from build123d import *

# Parameters (mm, degrees)
SKETCH_1_R          = 1.6
SKETCH_1_R_2        = 3.2
EXTRUDE_1_DEPTH     = 4
SKETCH_2_R          = 3.2
EXTRUDE_2_DEPTH     = 10
CUT_EXTRUDE_1_DEPTH = 10
CUT_EXTRUDE_2_DEPTH = 10


with BuildPart() as part:
    # 草图1 → 凸台-拉伸1 (new body)
    with BuildSketch(Plane.XY):
        Polygon((0, 0), (0, 26), (10, 26), (18, 18), (18, 8), (10, 0), align=None)
        with Locations((5, 21)):
            Circle(SKETCH_1_R, mode=Mode.SUBTRACT)
        with Locations((5, 13)):
            Circle(SKETCH_1_R_2, mode=Mode.SUBTRACT)
        with Locations((5, 5)):
            Circle(SKETCH_1_R, mode=Mode.SUBTRACT)
        with Locations((13, 13)):
            Circle(SKETCH_1_R, mode=Mode.SUBTRACT)
    extrude(amount=EXTRUDE_1_DEPTH)

    # 草图2 → 凸台-拉伸2 (add)
    with BuildSketch(Plane.XY.offset(4)):
        with BuildLine():
            Line((13.468501969, 16.468501969), (16.5, 19.5))
            Line((16.5, 19.5), (11.5, 24.5))
            Line((11.5, 24.5), (8.468501969, 21.468501969))
            ThreePointArc((8.468501969, 21.468501969), (7.104490226, 18.203373302), (3.589329863, 17.796875))
            ThreePointArc((3.589329863, 17.796875), (0, 13), (3.589329863, 8.203125))
            ThreePointArc((3.589329863, 8.203125), (7.104490226, 7.796626698), (8.468501969, 4.531498031))
            Line((8.468501969, 4.531498031), (11.5, 1.5))
            Line((11.5, 1.5), (16.5, 6.5))
            Line((16.5, 6.5), (13.468501969, 9.531498031))
            ThreePointArc((13.468501969, 9.531498031), (9.5, 13), (13.468501969, 16.468501969))
        make_face()
        with Locations((5, 13)):
            Circle(SKETCH_2_R, mode=Mode.SUBTRACT)
    extrude(amount=EXTRUDE_2_DEPTH)

    # 草图3 → 切除-拉伸1 (cut)
    with BuildSketch(Plane(origin=(-1.5, 1.5, 0), x_dir=(0, 0, -1), z_dir=(0.707106781, -0.707106781, 0))):
        Polygon((-4, 25.455844123), (-14, 25.455844123), (-14, 21.168658492), align=None)
    extrude(amount=-CUT_EXTRUDE_1_DEPTH, mode=Mode.SUBTRACT)

    # 草图4 → 切除-拉伸2 (cut)
    with BuildSketch(Plane(origin=(11.5, 11.5, 0), x_dir=(0, 0, -1), z_dir=(0.707106781, 0.707106781, 0))):
        Polygon((-4, -7.071067812), (-14, -2.783882181), (-14, -7.071067812), align=None)
    extrude(amount=-CUT_EXTRUDE_2_DEPTH, mode=Mode.SUBTRACT)


solid = part.part
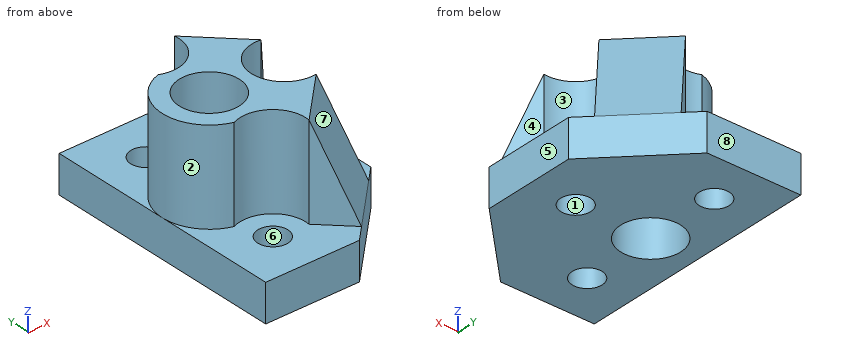
Part model, mm, in its own coordinate system. Face numbers are marked on the shaded views. A direction names the side the tool comes from. Coordinates: 2 decimals unless noted, no trailing zeros. Order: outer loops, then holes, each group sorted by start corner. A loop starts at its lowest first (then second) coordinate and runs counter-clockwise, first axis right, second up.
(1) Probe L1, parallel to Y at x = 5, z = 2; L2, parallel to Y at x = 5, z = 10.5; L3, parallel to Z at x = 10.25, y = 25. List the from-to ranges inside material, lowest first.
Check sheet entries:
L1: y = 0 to 3.4, 6.6 to 9.8, 16.2 to 19.4, 22.6 to 26
L2: y = 8.5 to 9.8, 16.2 to 17.5
L3: z = 0 to 4
(2) Pin check, flat tips, straight feed: pin 1 Ø5 at (x, y) = (13, 13) entering from +Z; pin 2 Ø6 at (x, y) = (5, 13) entering from +Z; pin 3 Ø6 at (x, z) = (15, 5.5) entering from -Y; pin 4 Ø2 at (x, z) = (9.5, 8.5) entering from -Y. Stop position of each tip, or through.
Check sheet entries:
pin 1: stops at z = 4
pin 2: passes through
pin 3: stops at y = 2.4
pin 4: stops at y = 2.69
(3) Slice it at A-A, the plane z = 1.25. Write the cut outline in (x, y).
Check sheet entries:
outline: (0, 0) - (10, 0) - (18, 8) - (18, 18) - (10, 26) - (0, 26) - close; hole circle Ø6.4 at (5, 13); hole circle Ø3.2 at (5, 5); hole circle Ø3.2 at (5, 21); hole circle Ø3.2 at (13, 13)
(4) Slice it at D-D, the plane z = 12.75. Write the cut outline in (x, y).
Check sheet entries:
outline: (3.59, 8.2) arc R3.5 cw to (8.47, 4.53) - (8.85, 4.15) - (13.85, 9.15) - (13.47, 9.53) arc R3.5 cw (long way) to (13.47, 16.47) - (13.85, 16.85) - (8.85, 21.85) - (8.47, 21.47) arc R3.5 cw to (3.59, 17.8) arc R5 ccw to start; hole circle Ø6.4 at (5, 13)
(5) Slice it at B-B, the plane x = 5. Write the cut outline in (y, z).
Check sheet entries:
outline: (0, 0) - (3.4, 0) - (3.4, 4) - (0, 4) - close; (6.6, 0) - (9.8, 0) - (9.8, 14) - (8.5, 14) - (8.5, 4) - (6.6, 4) - close; (16.2, 0) - (19.4, 0) - (19.4, 4) - (17.5, 4) - (17.5, 14) - (16.2, 14) - close; (22.6, 0) - (26, 0) - (26, 4) - (22.6, 4) - close
(6) Pull direction X, two halves, no side cores. Call the marked faces 6, 7 and 8: pulls with the +X half, pulls with the -X half, needs draft (parallel to the pull), parting line crosses it, or undercut.
Check sheet entries:
face 6: undercut
face 7: pulls with the +X half
face 8: needs draft
(7) Tool access for the marked faces 1, 2, 3, 4 and 5: list every direction of +Z, -Z, +X, -X, +Y, -Y with a clear straight run to the whole face (end or side of a thin tool).
Check sheet entries:
face 1: +Z, -Z
face 2: +Z, -X
face 3: +Z
face 4: +Z, +X
face 5: +Z, -Z, +X, +Y, -Y
(8) Slice it at C-C, the plane y = 10.5. Write the cut outline in (x, z).
Check sheet entries:
outline: (0, 0) - (3, 0) - (3, 14) - (0.67, 14) - (0.67, 4) - (0, 4) - close; (7, 0) - (18, 0) - (18, 4) - (10.55, 4) - (10.55, 14) - (7, 14) - close
